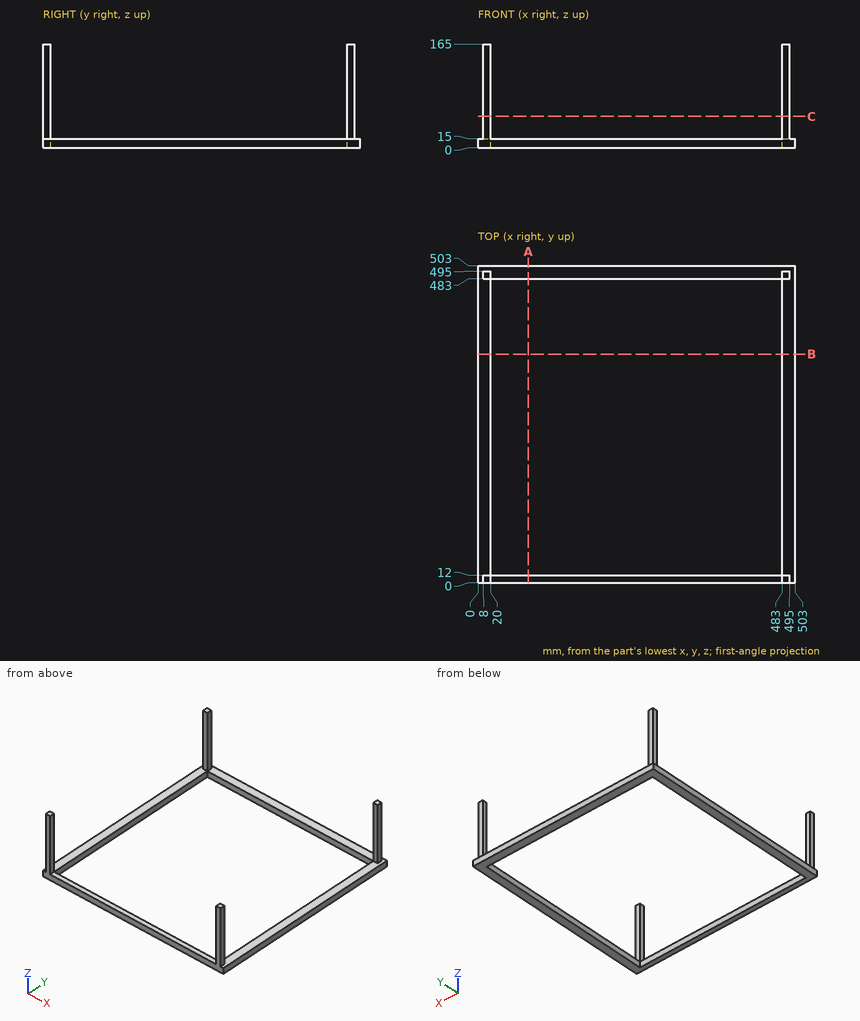
Source: three-view drawing plus pictorial views. Frame: mm from the lowest corner of the part. Coordinates: 2 decimals unless noted, no trailing zeros. Order: outer loops, then holes, each group sorted by start corner. A loop starts at its lowest first (then second) coordinate and runs counter-clockwise, first axis right, second up.
Item 1: Cut plane B-B (y = 363). Return loops of the section in (x, z).
Output values:
outline: (0, 0) - (20, 0) - (20, 15) - (0, 15) - close; (483, 0) - (503, 0) - (503, 15) - (483, 15) - close
Item 2: First-contact query: P1, Ø3.5, axis at x = 489.5, z = 92, coming from the +Y side; P2, Ø7.5, axis at y = 331.5, z = 8.5, coming from the -X side; P3, Ø6, axis at y = 7, z = 101.5, coming from the +X side; P4, Ø6, axis at y = 489.5, z = 78, coming from the -X side. Flat tips, straight axial feed; report the tip coordinate or a pass-through.
Output values:
P1: stops at y = 495
P2: stops at x = 0
P3: stops at x = 495
P4: stops at x = 8
Item 3: Cut plane A-A (x = 80). Return loops of the section in (y, z), plus the area to 3 significant figures.
Output values:
outline: (0, 0) - (12, 0) - (12, 15) - (0, 15) - close; (483, 0) - (503, 0) - (503, 15) - (483, 15) - close
area: 480 mm2
Item 4: Cut plane C-C (z = 50). Return loops of the section in (x, y), plus the area to 3 significant figures.
Output values:
outline: (8, 0) - (20, 0) - (20, 12) - (8, 12) - close; (8, 483) - (20, 483) - (20, 495) - (8, 495) - close; (483, 0) - (495, 0) - (495, 12) - (483, 12) - close; (483, 483) - (495, 483) - (495, 495) - (483, 495) - close
area: 576 mm2
Item 5: Material intervals for line 1 (X direction, y = 116, z = 7); line 2 (Y direction, x = 200.5, z = 7), sorted ascending.
Output values:
line 1: x = 0 to 20, 483 to 503
line 2: y = 0 to 12, 483 to 503
